Work out the finished part from the listing and answer in its coordinate system (mm). Round coordinates to 2 decimals unless told otherwise and drop trailing zeros. Write each loop counter-clockwise with the first axis right and the second up, starting at its lowest first coordinate (ties: lowest second). Pieces come first, ordered by that corner, then holes. Notation, with made-up numbers: M 25.5,-39.75 L 44.5,-39.75 A23 cw 44.5,-14.75 Z; hole C 77,-39 d8. An arc over 180 degrees is marked long. One line per item, written item: value. Start each with the question number.
Q1. Consider probe 1 along X at (y, z) = (-16, 81.5); probe 2 along X at (y, z) = (-8, 276.5); probe 3 along Z at (x, y) = (-390.5, -10.5). Determine where each line is inside the solid, lowest interval first.
Q2. Given pin 1 Ø6 at (y, z) = (-2.5, 253.5) entering from -X; pin 2 Ø6 at (x, y) = (140, -13) entering from +Z, each flat-ended and moving along its own axis, determine where each tip first touches the part or whether it passes through.
Q3. Find section A-A (y = -14.5). Write down the section's boundary in (x, z), and give its area (3 significant figures).
from build123d import *

# Parameters (mm, degrees)
F1_DEPTH = 18
F2_R     = 10


with BuildPart() as f1:
    # F0 (on Front) → F1 (new body)
    with BuildSketch(Plane.XZ):
        with BuildLine():
            ThreePointArc((512.5, 205), (477.352814, 289.852814), (392.5, 325))
            Line((392.5, 325), (-392.5, 325))
            ThreePointArc((-392.5, 325), (-477.352814, 289.852814), (-512.5, 205))
            Line((-512.5, 205), (-512.5, -325))
            Line((-512.5, -325), (512.5, -325))
            Line((512.5, -325), (512.5, 205))
        make_face()
    extrude(amount=F1_DEPTH)

    # F2
    f2_edges = [f1.edges().sort_by_distance(p)[0] for p in [
        (0, -18, 325),
    ]]
    fillet(f2_edges, radius=F2_R)


solid = f1.part
The answers:
1. probe 1: -508.5 to 508.5
1. probe 2: -488.87 to 488.87
1. probe 3: -325 to 324.68
2. pin 1: x = -503.54
2. pin 2: z = 324.8
3. outline: M -510.1,-325 L 510.1,-325 L 510.1,205 A117.6 ccw 392.5,322.6 L -392.5,322.6 A117.6 ccw -510.1,205 Z
3. area: 655,000 mm2
